The drawing under review shows one solid part. Ordinate dimensions are in mm from its lowest x, y, z. Coordinates: 2 decimals unless noted, no trailing zeros. Write each loop counter-clockwise with the first axis right and the second up, starting at its lowest first coordinate (ties: lowest second). Pieces come first, ordered by that corner, then holes.
Q1. Add section C-C, the plane y = 1.65. Give the number of separate pieces and of enclosed holes in the cut face, plus the area to 3 significant figures.
Q2. Clearance check with a flat-ended pin moving along its axis: pin 1 Ø1.5 at (x, y) = (44.5, 1) entering from -Z. State where the tip first meets the part, or that it passes through.
Q3. Add section A-A, the plane x = 15. Give the boundary of the cut face in (y, z).
Q4. To check wall thickness, follow probe 1 along X at (y, z) = (2.45, 32); probe 2 along X at (y, z) = (1.3, 5); probe 3 along Z at (x, y) = (15, 1.2). State the ranges of each line that lie inside material, in increasing order.
Q5. Add section B-B, the plane z = 5. Give the boundary of the cut face in (x, y), plus the area to 3 significant figures.
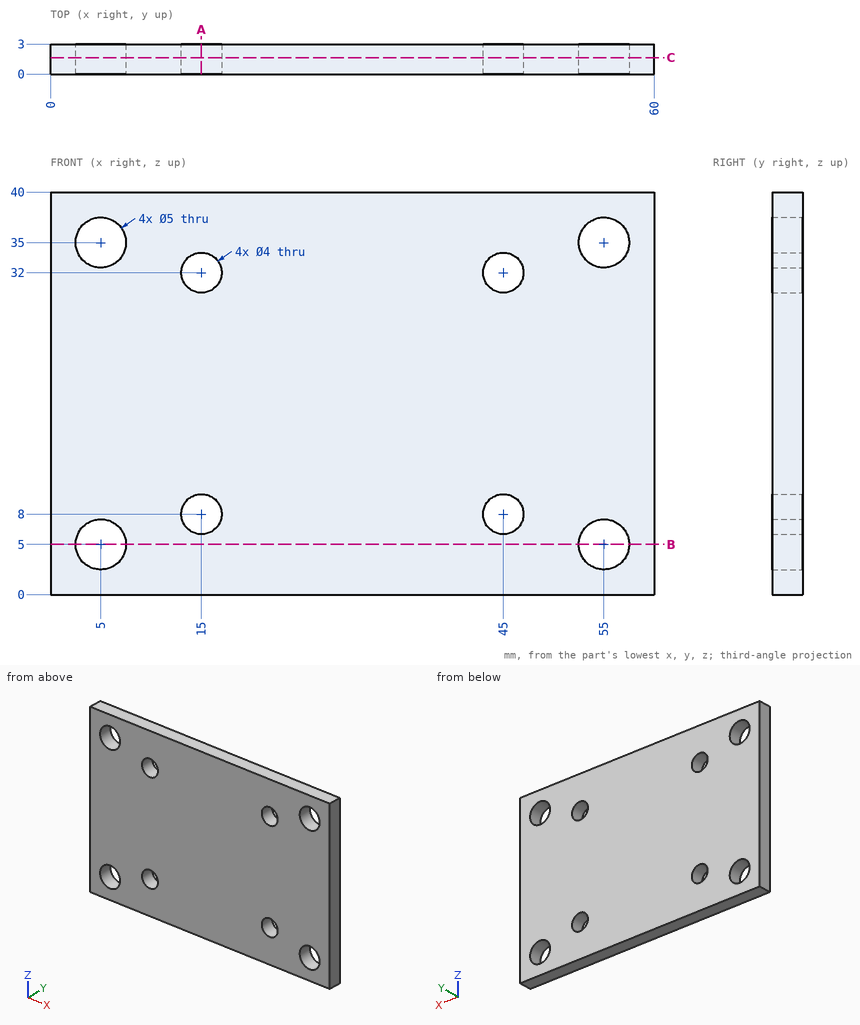
Here are the results:
1. separate pieces: 1
1. enclosed holes: 8
1. area: 2,270 mm2
2. pin 1: stops at z = 0
3. outline: (0, 0) - (3, 0) - (3, 6) - (0, 6) - close; (0, 10) - (3, 10) - (3, 30) - (0, 30) - close; (0, 34) - (3, 34) - (3, 40) - (0, 40) - close
4. probe 1: x = 0 to 13, 17 to 43, 47 to 60
4. probe 2: x = 0 to 2.5, 7.5 to 52.5, 57.5 to 60
4. probe 3: z = 0 to 6, 10 to 30, 34 to 40
5. outline: (0, 0) - (2.5, 0) - (2.5, 3) - (0, 3) - close; (7.5, 0) - (52.5, 0) - (52.5, 3) - (7.5, 3) - close; (57.5, 0) - (60, 0) - (60, 3) - (57.5, 3) - close
5. area: 150 mm2
